CAD build for the part. Positions are in the model's coordinates, mm. A direction names the side the tool comes from. Round coordinates to 2 decimals unless told otherwise and drop trailing zeros. Write each loop counter-clockwise with the first axis right and the second up, starting at its lowest first coordinate (ties: lowest second). Pieces come first, ordered by that corner, then holes. Notation, with made-up numbers: (64.25, 10.25) - (97.25, 10.25) arc R11 cw to (97.25, 14.25) - close; hole circle Ø3 at (58.5, 43). An arc over 180 degrees is marked (long way). Answer in a Markdown table with one row per item.
```python
from build123d import *

# Parameters (mm, degrees)
BOSS_EXTRUDE1_DEPTH = 2.286
CUT_EXTRUDE1_DEPTH  = 126.744366856
SKETCH3_R           = 2.4638
CUT_EXTRUDE2_DEPTH  = 126.744366999


with BuildPart() as part:
    # Sketch1 → Boss-Extrude1 (new body)
    with BuildSketch(Plane(origin=(0, 0, 0), x_dir=(1, 0, 0), z_dir=(0, 1, 0))):
        Polygon((25.4, 63.5), (63.5, 25.4), (88.9, 25.4), (88.9, 0), (0, 0), (0, 88.9), (25.4, 88.9), align=None)
    extrude(amount=BOSS_EXTRUDE1_DEPTH)

    # Sketch2 → Cut-Extrude1 (cut, through all)
    with BuildSketch(Plane(origin=(0, 2.286, 0), x_dir=(1, 0, 0), z_dir=(0, 1, 0))):
        with BuildLine():
            add(Edge.make_bspline(
                [(31.65582917, 44.824706507), (31.72721015, 44.868168803), (31.870288171, 44.955285838), (32.115061475, 45.030799557), (32.37800112, 45.066201469), (32.558110333, 45.05330926), (32.651195267, 45.046646245)],
                knots=[0, 0, 0, 0, 0.959878879, 1.924007909, 2.927075513, 4, 4, 4, 4], degree=3))
            Line((32.651195267, 45.046646245), (36.831060331, 42.050459784))
            add(Edge.make_bspline(
                [(36.831060331, 42.050459784), (36.874582097, 41.996816639), (36.963947184, 41.886668896), (37.019807322, 41.663032648), (36.998735396, 41.406700154), (36.946797609, 41.231360456), (36.918491136, 41.135799046)],
                knots=[0, 0, 0, 0, 0.847093379, 1.739372747, 2.767941704, 4, 4, 4, 4], degree=3))
            add(Edge.make_bspline(
                [(36.918491136, 41.135799046), (36.907659111, 41.100371643), (36.884120075, 41.023384482), (36.811679346, 40.91436251), (36.720386672, 40.794599967), (36.64589915, 40.716950958), (36.605757869, 40.675105953)],
                knots=[0, 0, 0, 0, 0.786237394, 1.708569685, 2.765149586, 4, 4, 4, 4], degree=3))
            add(Edge.make_bspline(
                [(36.605757869, 40.675105953), (36.534614921, 40.6177911), (36.384603144, 40.496937196), (36.196750402, 40.452821185), (36.097986651, 40.429627152)],
                knots=[0, 0, 0, 0, 0.948498166, 2, 2, 2, 2], degree=3))
            Line((36.097986651, 40.429627152), (35.778527937, 40.480068002))
            Line((35.778527937, 40.480068002), (31.58521198, 42.642299085))
            Line((31.58521198, 42.642299085), (25.855131474, 36.912218579))
            Line((25.855131474, 36.912218579), (34.315743301, 35.546952919))
            add(Edge.make_bspline(
                [(34.315743301, 35.546952919), (34.378329612, 35.529086939), (34.490251228, 35.497137631), (34.593189369, 35.443023199), (34.638564738, 35.419169433)],
                knots=[0, 0, 0, 0, 1.11839541, 2, 2, 2, 2], degree=3))
            add(Edge.make_bspline(
                [(34.638564738, 35.419169433), (34.683076904, 35.345786024), (34.768509207, 35.204941079), (34.807974339, 35.045116744), (34.826877243, 34.968564511)],
                knots=[0, 0, 0, 0, 1.042045342, 2, 2, 2, 2], degree=3))
            Line((34.826877243, 34.968564511), (36.050908525, 26.447423665))
            Line((36.050908525, 26.447423665), (42.107173191, 32.503688331))
            Line((42.107173191, 32.503688331), (40.361919797, 35.923577928))
            add(Edge.make_bspline(
                [(40.361919797, 35.923577928), (40.351753136, 35.974985176), (40.330871112, 36.080574163), (40.3439389, 36.246210329), (40.367095634, 36.421433735), (40.407855126, 36.536130678), (40.429174263, 36.596122589)],
                knots=[0, 0, 0, 0, 0.913209557, 1.875705789, 2.888893945, 4, 4, 4, 4], degree=3))
            add(Edge.make_bspline(
                [(40.429174263, 36.596122589), (40.509009346, 36.672362665), (40.651215954, 36.808165651), (40.849356719, 36.972690697), (41.015708613, 37.074515143), (41.12005501, 37.088251343), (41.162247943, 37.093805637)],
                knots=[0, 0, 0, 0, 1.466202942, 2.611680716, 3.438626887, 4, 4, 4, 4], degree=3))
            add(Edge.make_bspline(
                [(41.162247943, 37.093805637), (41.243888372, 37.10647383), (41.393272638, 37.129653873), (41.601794633, 37.125883922), (41.776610643, 37.083447982), (41.862114812, 37.017157534), (41.902047069, 36.986198492)],
                knots=[0, 0, 0, 0, 1.278063421, 2.338578655, 3.224081066, 4, 4, 4, 4], degree=3))
            Line((41.902047069, 36.986198492), (44.777175492, 32.913940573))
            add(Edge.make_bspline(
                [(44.777175492, 32.913940573), (44.794644521, 32.874178054), (44.836759395, 32.778317344), (44.821784918, 32.589132207), (44.777454045, 32.347784995), (44.719281585, 32.170283543), (44.686381963, 32.069897025)],
                knots=[0, 0, 0, 0, 0.592454987, 1.428308758, 2.545571737, 4, 4, 4, 4], degree=3))
            Line((44.686381963, 32.069897025), (35.876046913, 23.259561975))
            add(Edge.make_bspline(
                [(35.876046913, 23.259561975), (35.802583462, 23.210319908), (35.662434184, 23.11637877), (35.410146741, 23.084728901), (35.156417578, 23.137802986), (35.012256253, 23.238737342), (34.934484389, 23.293189208)],
                knots=[0, 0, 0, 0, 1.024762661, 1.954982311, 2.896757927, 4, 4, 4, 4], degree=3))
            add(Edge.make_bspline(
                [(34.934484389, 23.293189208), (34.862211763, 23.371249908), (34.725830705, 23.518553272), (34.655031564, 23.706083117), (34.621751121, 23.79423498)],
                knots=[0, 0, 0, 0, 1.059863105, 2, 2, 2, 2], degree=3))
            Line((34.621751121, 23.79423498), (33.269936354, 33.337643709))
            Line((33.269936354, 33.337643709), (33.212770058, 33.260301073))
            Line((33.212770058, 33.260301073), (23.370078955, 34.945025448))
            add(Edge.make_bspline(
                [(23.370078955, 34.945025448), (23.325591172, 34.969657633), (23.229222166, 35.023015636), (23.143726057, 35.092543958), (23.097698367, 35.129975229)],
                knots=[0, 0, 0, 0, 0.923279883, 2, 2, 2, 2], degree=3))
            add(Edge.make_bspline(
                [(23.097698367, 35.129975229), (23.056477465, 35.174430553), (22.978267135, 35.258777702), (22.896457595, 35.403808998), (22.845356477, 35.551168549), (22.835942364, 35.750716315), (22.882407019, 36.001780496), (22.991741999, 36.170711674), (23.047257518, 36.256487535)],
                knots=[0, 0, 0, 0, 0.874892655, 1.659974428, 2.393902707, 3.109661626, 4.532412633, 6, 6, 6, 6], degree=3))
            Line((23.047257518, 36.256487535), (31.65582917, 44.824706507))
        make_face()
    extrude(amount=-CUT_EXTRUDE1_DEPTH, mode=Mode.SUBTRACT)

    # Sketch3 → Cut-Extrude2 (cut, through all)
    with BuildSketch(Plane(origin=(0, 2.286, 0), x_dir=(1, 0, 0), z_dir=(0, 1, 0))):
        with Locations(Location((76.2, 12.7, 0), (0, 0, 270))):
            Circle(SKETCH3_R)
        with Locations(Location((12.7, 12.7, 0), (0, 0, 270))):
            Circle(SKETCH3_R)
        with Locations(Location((12.7, 76.2, 0), (0, 0, 270))):
            Circle(SKETCH3_R)
        with Locations(Location((12.7, 38.1, 0), (0, 0, 270))):
            Circle(SKETCH3_R)
        with Locations(Location((38.1, 12.7, 0), (0, 0, 270))):
            Circle(SKETCH3_R)
    extrude(amount=-CUT_EXTRUDE2_DEPTH, mode=Mode.SUBTRACT)


solid = part.part
```
Q1. Flat gauge pins, fed straight in: pin 1 (0.7 mm diameter, centred on y = 1.5, z = -74, fed in from +X); pin 2 (1.1 mm diameter, centred on x = 74, y = 0.5, fed in from -Z); pin 3 (4.5 mm diameter, centred on x = 12.7, z = -12.7, fed in from +Y). Where does each tip first touch, or does it go through?
Computed:
| item | result |
|---|---|
| pin 1 | stops at x = 25.4 |
| pin 2 | stops at z = -25.4 |
| pin 3 | passes through |
Q2. Saw through at A-A on x = 76.2. List the corners of the cut face in (y, z), then the cut area to 3 significant figures.
Computed:
| item | result |
|---|---|
| outline | (0, -25.4) - (2.29, -25.4) - (2.29, -15.16) - (0, -15.16) - close; (0, -10.24) - (2.29, -10.24) - (2.29, 0) - (0, 0) - close |
| area | 46.8 mm2 |
Q3. Saw through at D-D on x = 12.7. List the corners of the cut face in (y, z).
Computed:
| item | result |
|---|---|
| outline | (0, -88.9) - (2.29, -88.9) - (2.29, -78.66) - (0, -78.66) - close; (0, -73.74) - (2.29, -73.74) - (2.29, -40.56) - (0, -40.56) - close; (0, -35.64) - (2.29, -35.64) - (2.29, -15.16) - (0, -15.16) - close; (0, -10.24) - (2.29, -10.24) - (2.29, 0) - (0, 0) - close |
Q4. Drill centre lines: line 1 (X direction, y = 0.8, z = -12.7); line 2 (Z direction, x = 32.5, y = 1.4); line 3 (Z direction, x = 12, y = 1.35). Where is each one in solid material? Low to high.
Computed:
| item | result |
|---|---|
| line 1 | x = 0 to 10.24, 15.16 to 35.64, 40.56 to 73.74, 78.66 to 88.9 |
| line 2 | z = -56.4 to -45.06, -42.17 to -35.84, -33.38 to 0 |
| line 3 | z = -88.9 to -78.56, -73.84 to -40.46, -35.74 to -15.06, -10.34 to 0 |
Q5. Saw through at B-B on z = -12.7. List the corners of the cut face in (x, y).
Computed:
| item | result |
|---|---|
| outline | (0, 0) - (10.24, 0) - (10.24, 2.29) - (0, 2.29) - close; (15.16, 0) - (35.64, 0) - (35.64, 2.29) - (15.16, 2.29) - close; (40.56, 0) - (73.74, 0) - (73.74, 2.29) - (40.56, 2.29) - close; (78.66, 0) - (88.9, 0) - (88.9, 2.29) - (78.66, 2.29) - close |
Q6. 3-axis set-ups, long thin cutter, end or side, ignore diameter. For faces 1 (the flat face through (34.71, 1.16, -43.57)), 2 (the flat face through (0, 1, -44)), 3 (the flat face through (25.4, 1, -76)): which of +Z, -Z, +X, -X, +Y, -Y reach the whole face in a straight line?
Computed:
| item | result |
|---|---|
| face 1 | +Y, -Y |
| face 2 | +Z, -Z, -X, +Y, -Y |
| face 3 | -Z, +X, +Y, -Y |
Q7. Saw through at C-C on z = -76.2. List the corners of the cut face in (x, y), then the cut area to 3 significant figures.
Computed:
| item | result |
|---|---|
| outline | (0, 0) - (10.24, 0) - (10.24, 2.29) - (0, 2.29) - close; (15.16, 0) - (25.4, 0) - (25.4, 2.29) - (15.16, 2.29) - close |
| area | 46.8 mm2 |
Q8. Pull direction Z, two halves, no side cores. Call faces 4 (the flat face through (35, 0, -35)), 5 (the flat face through (45, 1, 0)), 6 (the flat face through (35.43, 1.16, -30.77)): released by +Z, released by -Z, zero draft, split by the parting line, or undercut.
Computed:
| item | result |
|---|---|
| face 4 | zero draft |
| face 5 | released by +Z |
| face 6 | undercut |
